```python
from build123d import *

# Parameters (mm, degrees)
SKETCH1_W           = 40
SKETCH1_H           = 30
BOSS_EXTRUDE1_DEPTH = 15
CUT_EXTRUDE1_DEPTH  = 15
SKETCH3_R           = 1.375
CUT_EXTRUDE2_DEPTH  = 15


with BuildPart() as part:
    # Sketch1 → Boss-Extrude1 (new body)
    with BuildSketch(Plane(origin=(0, 0, 0), x_dir=(1, 0, 0), z_dir=(0, 1, 0))):
        with Locations((-14.816176471, 3.033088235)):
            Rectangle(SKETCH1_W, SKETCH1_H)
    extrude(amount=BOSS_EXTRUDE1_DEPTH)

    # Sketch2 → Cut-Extrude1 (cut)
    with BuildSketch(Plane(origin=(0, 15, 0), x_dir=(1, 0, 0), z_dir=(0, 1, 0))):
        Polygon((-28.816176471, 3.033088235), (-28.816176471, 18.033088235), (-34.816176471, 18.033088235), align=None)
        with BuildLine():
            Line((-0.816176471, 18.033088235), (-28.816176471, 18.033088235))
            Line((-28.816176471, 18.033088235), (-28.816176471, 3.033088235))
            Line((-28.816176471, 3.033088235), (-21.816176471, 3.033088235))
            ThreePointArc((-21.816176471, 3.033088235), (-14.816176471, 10.033088235), (-7.816176471, 3.033088235))
            Line((-7.816176471, 3.033088235), (-0.816176471, 3.033088235))
            Line((-0.816176471, 3.033088235), (-0.816176471, 18.033088235))
        make_face()
        Polygon((5.183823529, 18.033088235), (-0.816176471, 18.033088235), (-0.816176471, 3.033088235), align=None)
        Polygon((5.183823529, 18.033088235), (-0.816176471, 3.033088235), (-0.816176471, -11.966911765), (5.183823529, -11.966911765), align=None)
        Polygon((-0.816176471, -11.966911765), (-0.816176471, 3.033088235), (-6.816176471, -11.966911765), align=None)
        Polygon((-22.816176471, -11.966911765), (-28.816176471, 3.033088235), (-28.816176471, -11.966911765), align=None)
        Polygon((-28.816176471, -11.966911765), (-28.816176471, 3.033088235), (-34.816176471, 18.033088235), (-34.816176471, -11.966911765), align=None)
        with BuildLine():
            ThreePointArc((-7.816176471, 3.033088235), (-14.816176471, 10.033088235), (-21.816176471, 3.033088235))
            Line((-21.816176471, 3.033088235), (-7.816176471, 3.033088235))
        make_face()
        with BuildLine():
            Line((-7.816176471, 3.033088235), (-21.816176471, 3.033088235))
            ThreePointArc((-21.816176471, 3.033088235), (-14.816176471, -3.966911765), (-7.816176471, 3.033088235))
        make_face()
    extrude(amount=-CUT_EXTRUDE1_DEPTH, mode=Mode.SUBTRACT)

    # Sketch3 → Cut-Extrude2 (cut)
    with BuildSketch(Plane(origin=(0, 0, -3.033088235), x_dir=(-1, 0, 0), z_dir=(0, 0, -1))):
        with Locations((3.566176471, 7.5)):
            Circle(SKETCH3_R)
        with Locations((26.066176471, 7.5)):
            Circle(SKETCH3_R)
    extrude(amount=-CUT_EXTRUDE2_DEPTH, mode=Mode.SUBTRACT)


solid = part.part
```
Model file for the job. Use its own axes, mm. Round coordinates to 2 decimals unless told otherwise and drop trailing zeros. Loops run counter-clockwise (first coordinate to the right, second up) from the corner with the lowest first, then second, coordinate; pieces in that order, holes last. Notation, with made-up numbers: M 55.25,38 L 104.25,38 A4 cw 104.25,43 Z; hole C 24.5,69 d7. An arc over 180 degrees is marked long. Put each result on its own line as item: value. Start each with the question number.
Item 1: Cut at A-A (z = 1). List the corners of the cut face in (x, y) (3 decimals), then the cut area to 3 significant figures.
Item 2: Cut at B-B (y = 1). List the corners of the cut face in (x, z).
Item 3: Drill centre lines: line 1 along X through (y, z) = (9, 0.25); line 2 along X through (y, z) = (10.25, 3); line 3 along Z through (x, y) = (-16.25, 12). Where is each one in solid material? Low to high.
Item 4: Cut at C-C (z = 4.25). List the corners of the cut face in (x, y) (3 decimals), then the cut area to 3 significant figures.
Item 5: Mould opens along X. For faces 1 (the face through (-14.97, 7.605, 3.965)), 2 (the face through (-5.1, 7.6, -3.033)), 3 (the face through (-25.774, 5.938, 4.572)) say: released by +X, released by -X, zero draft, split by the parting line, or undercut.
Item 6: Cut at D-D (y = 7.5). List the corners of the cut face in (x, z).
Item 7: Drop flat-ended pins along their axis: P1, Ø6, axis at y = 13, z = 6.5, coming from the +X side; P2, Ø1, axis at y = 10, z = 6, coming from the +X side. Give the stop position or say it passes through.
Answer block:
1. outline: M -27.203,0 L -20.538,0 L -20.538,15 L -27.203,15 L -27.203,8.274 A1.375 cw long -27.203,6.726 Z; M -9.095,0 L -2.429,0 L -2.429,6.726 A1.375 cw long -2.429,8.274 L -2.429,15 L -9.095,15 Z
1. area: 189 mm2
2. outline: M -28.82,-3.03 L -21.82,-3.03 A7 cw -7.82,-3.03 L -0.82,-3.03 L -6.82,11.97 L -22.82,11.97 Z
3. line 1: -27.5 to -21, -8.63 to -2.13
3. line 2: -26.4 to -18.37, -11.27 to -3.23
3. line 3: 3.82 to 11.97
4. outline: M -25.903,0 L -3.729,0 L -3.729,6.135 A1.375 cw -3.729,8.865 L -3.729,15 L -25.903,15 L -25.903,8.865 A1.375 cw -25.903,6.135 Z
4. area: 328 mm2
5. face 1: undercut
5. face 2: zero draft
5. face 3: released by -X
6. outline: M -28.82,-3.03 L -27.44,-3.03 L -27.44,0.4 Z; M -24.69,-3.03 L -21.82,-3.03 A7 cw -7.82,-3.03 L -4.94,-3.03 L -4.94,7.28 L -6.82,11.97 L -22.82,11.97 L -24.69,7.28 Z; M -2.19,-3.03 L -0.82,-3.03 L -2.19,0.4 Z
7. P1: x = -3.43
7. P2: x = -4.23
